The listing builds one solid part. Answer for the finished solid, in the listing's coordinates (mm). Face numbers are marked on the shaded views. A direction names the side the tool comes from. Coordinates: 2 decimals unless noted, no trailing zeros. Order: outer loops, then holes, each group sorted by start corner. A loop starts at its lowest first (then second) coordinate and runs counter-clockwise, first axis right, second up. Notation, with made-up numbers: (-38.75, -13) -> (0.25, -13) arc R22 cw to (0.25, -2) -> close; hole circle Ø9 at (-5, -38.5). An arc over 180 degrees is marked (long way). One line per question, with ' | ' between items.
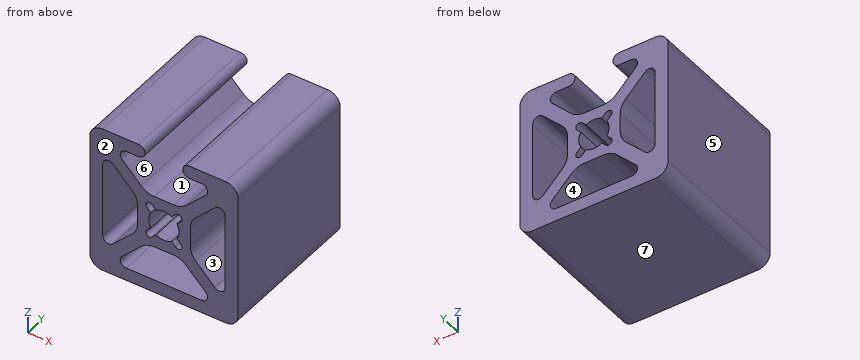
Autodesk Inventor part; units mm, degrees
ref_plane "YZ Plane" through (0, 0, 0) normal (1, 0, 0) x (0, 1, 0)
ref_plane "XZ Plane" through (0, 0, 0) normal (0, 1, 0) x (-1, 0, 0)
ref_plane "XY Plane" through (0, 0, 0) normal (0, 0, 1) x (1, 0, 0)
sketch "Sketch1" plane through (0, 0, 0) normal (0, 1, 0) x (-1, 0, 0)
  arc A0 (4.5172, -1.6395) -> (5.4471, -3.8845) centre (7.6922, -1.6395) ccw
  line L0 (8.7558, -7.1932) -> (5.4471, -3.8845)
  arc A1 (8.7558, -7.1932) -> (10.4902, -6.4748) centre (9.4742, -6.4748) ccw
  line L1 (10.4902, 6.4748) -> (10.4902, -6.4748)
  arc A2 (10.4902, 6.4748) -> (8.7558, 7.1932) centre (9.4742, 6.4748) ccw
  line L2 (5.4471, 3.8845) -> (8.7558, 7.1932)
  arc A3 (5.4471, 3.8845) -> (4.5172, 1.6395) centre (7.6922, 1.6395) ccw
  line L3 (4.5172, -1.6395) -> (4.5172, 1.6395)
  arc A4 (6.4748, -10.4902) -> (7.1932, -8.7558) centre (6.4748, -9.4742) ccw
  line L4 (3.8845, -5.4471) -> (7.1932, -8.7558)
  arc A5 (3.8845, -5.4471) -> (1.6394, -4.5172) centre (1.6394, -7.6922) ccw
  line L5 (-1.6395, -4.5172) -> (1.6394, -4.5172)
  arc A6 (-1.6395, -4.5172) -> (-3.8846, -5.4471) centre (-1.6395, -7.6922) ccw
  line L6 (-7.1932, -8.7558) -> (-3.8846, -5.4471)
  arc A7 (-7.1932, -8.7558) -> (-6.4748, -10.4902) centre (-6.4748, -9.4742) ccw
  line L7 (6.4748, -10.4902) -> (-6.4748, -10.4902)
  arc A8 (-10.4902, -6.4749) -> (-8.7557, -7.1933) centre (-9.4742, -6.4749) ccw
  line L8 (-5.4471, -3.8846) -> (-8.7557, -7.1933)
  arc A9 (-5.4471, -3.8846) -> (-4.5171, -1.6396) centre (-7.6921, -1.6396) ccw
  line L9 (-4.5171, 1.6394) -> (-4.5171, -1.6396)
  arc A10 (-4.5171, 1.6394) -> (-5.4471, 3.8844) centre (-7.6921, 1.6394) ccw
  line L10 (-8.7557, 7.1931) -> (-5.4471, 3.8844)
  arc A11 (-8.7557, 7.1931) -> (-10.4902, 6.4747) centre (-9.4742, 6.4747) ccw
  line L11 (-10.4902, -6.4749) -> (-10.4902, 6.4747)
  arc A12 (1.3405, 2.2319) -> (-1.3405, 2.2319) centre (0, 0) ccw
  line L12 (-1.9692, 2.8605) -> (-1.3405, 2.2319)
  arc A13 (-1.9692, 2.8605) -> (-2.8605, 1.9692) centre (-2.4696, 2.4696) ccw
  line L13 (-2.2319, 1.3405) -> (-2.8605, 1.9692)
  arc A14 (-2.2319, 1.3405) -> (-2.2319, -1.3405) centre (0, 0) ccw
  line L14 (-2.8605, -1.9692) -> (-2.2319, -1.3405)
  arc A15 (-2.8605, -1.9692) -> (-1.9692, -2.8605) centre (-2.4696, -2.4696) ccw
  line L15 (-1.3405, -2.2319) -> (-1.9692, -2.8605)
  arc A16 (-1.3405, -2.2319) -> (1.3405, -2.2319) centre (0, 0) ccw
  line L16 (1.9692, -2.8605) -> (1.3405, -2.2319)
  arc A17 (1.9692, -2.8605) -> (2.8605, -1.9692) centre (2.4696, -2.4696) ccw
  line L17 (2.2319, -1.3405) -> (2.8605, -1.9692)
  arc A18 (2.2319, -1.3405) -> (2.2319, 1.3405) centre (0, 0) ccw
  line L18 (2.8605, 1.9692) -> (2.2319, 1.3405)
  arc A19 (2.8605, 1.9692) -> (1.9692, 2.8605) centre (2.4696, 2.4696) ccw
  line L19 (1.3405, 2.2319) -> (1.9692, 2.8605)
  arc A20 (-4.3561, 10.4904) -> (-4.3452, 12.7001) centre (-4.3451, 11.5952) ccw
  line L20 (-4.3561, 10.4904) -> (-6.4749, 10.4903)
  arc A21 (-6.4749, 10.4903) -> (-7.1933, 8.7559) centre (-6.4749, 9.4743) ccw
  line L21 (-7.1933, 8.7559) -> (-3.8846, 5.4472)
  arc A22 (-3.8846, 5.4472) -> (-1.6396, 4.5173) centre (-1.6396, 7.6923) ccw
  line L22 (-1.6396, 4.5173) -> (1.6397, 4.5173)
  arc A23 (1.6397, 4.5173) -> (3.8848, 5.4472) centre (1.6397, 7.6923) ccw
  line L23 (3.8848, 5.4472) -> (7.1935, 8.7559)
  arc A24 (7.1935, 8.7559) -> (6.475, 10.4903) centre (6.475, 9.4743) ccw
  line L24 (6.475, 10.4903) -> (4.3616, 10.4903)
  arc A25 (4.3616, 12.7001) -> (4.3616, 10.4903) centre (4.3616, 11.5952) ccw
  line L25 (4.3616, 12.7001) -> (10.5011, 12.7001)
  arc A26 (12.7109, 10.4903) -> (10.5011, 12.7001) centre (10.5011, 10.4903) ccw
  line L26 (12.7109, 10.4903) -> (12.7109, -10.5917)
  arc A27 (10.6027, -12.6999) -> (12.7109, -10.5917) centre (10.6027, -10.5917) ccw
  line L27 (10.6027, -12.6999) -> (-10.5992, -12.6999)
  arc A28 (-12.7074, -10.5917) -> (-10.5992, -12.6999) centre (-10.5992, -10.5917) ccw
  line L28 (-12.7074, -10.5917) -> (-12.7074, 10.5919)
  arc A29 (-10.5809, 12.7) -> (-12.7074, 10.5919) centre (-10.5992, 10.5919) ccw
  line L29 (-10.5809, 12.7) -> (-4.3452, 12.7001)
  point P0 (0, 0)
  dimension "d100" = 8.1828
  dimension "d103" = 25.4
extrude "Extrusion1" add sketch "Sketch1" along normal mid plane 25.4
properties part number "1001-S-BLACK-FB" material "6105-T5"
Item 1: Section B-B, the plane y = -10 is taken. Count the separate pieces of the cut face and the enclosed holes in it, plus the area to 3 significant figures.
Computed values:
separate pieces: 1 | enclosed holes: 4 | area: 326 mm^2
Item 2: For the marked faces 1, 2 and 3, determine the directions among +Z, -Z, +X, -X, +Y, -Y from which every point of the face is accessible in a straight line to the end or side of a thin tool.
Computed values:
face 1: +Z, +Y, -Y | face 2: +Z, -Z, +X, -X, -Y | face 3: +Y, -Y
Item 3: Find the intervals of material crossed by L1, parallel to Z at x = 4, y = -11; L2, parallel to X at y = -2.25, z = -3.75; L3, parallel to Z at x = 1.25, y = 4.75, in increasing order.
Computed values:
L1: z = -12.7 to -10.49, -5.56 to 5.56, 10.55 to 12.64 | L2: x = -12.71 to -10.49, -5.32 to 5.32, 10.49 to 12.71 | L3: z = -12.7 to -10.49, -4.52 to -2.28, 2.28 to 4.52
Item 4: Each of these flat-tipped pins is pushed along its axis until it touches: pin 1 Ø1 at (x, z) = (-2.47, -2.47) entering from +Y; pin 2 Ø3.5 at (x, y) = (0, 4) entering from +Z. Where does it stop, or does it pass through?
Computed values:
pin 1: passes through | pin 2: stops at z = 4.52
Item 5: Section A-A, the plane x = 0.5 is taken. Give the vertices of the cut face in (y, z).
Computed values:
outline: (-12.7, -12.7) -> (12.7, -12.7) -> (12.7, -10.49) -> (-12.7, -10.49) -> close; (-12.7, -4.52) -> (12.7, -4.52) -> (12.7, -2.56) -> (-12.7, -2.56) -> close; (-12.7, 2.56) -> (12.7, 2.56) -> (12.7, 4.52) -> (-12.7, 4.52) -> close
Item 6: Section C-C, the plane x = -8 is taken. Give the vertices of the cut face in (y, z), plus the area to 3 significant figures.
Computed values:
outline: (-12.7, -12.7) -> (12.7, -12.7) -> (12.7, -6.44) -> (-12.7, -6.44) -> close; (-12.7, 6.44) -> (12.7, 6.44) -> (12.7, 12.7) -> (-12.7, 12.7) -> close | area: 318 mm^2
Item 7: Determine the mould class of the marked faces 4, 5, 6 and 7 for opening direction X: pulls with the +X half, pulls with the -X half, needs draft (parallel to the pull), parting line crosses it, or undercut.
Computed values:
face 4: undercut | face 5: pulls with the -X half | face 6: undercut | face 7: needs draft
